from build123d import *

# Parameters (mm, degrees)
BOX023_W     = 2
BOX023_H     = 10
BOX023_DEPTH = 8.5
BOX025_W     = 6
BOX025_H     = 14
BOX025_DEPTH = 1


with BuildPart() as control_button_rec_c:
    # Box023 → Box023 (new body)
    with BuildSketch(Plane(origin=(57.3, 93.3, 9.6), x_dir=(1, 0, 0), z_dir=(0, 0, 1))):
        with Locations((1, 5)):
            Rectangle(BOX023_W, BOX023_H)
    extrude(amount=BOX023_DEPTH)


with BuildPart() as control_button_rec:
    # Box025 → Box025 (new body)
    with BuildSketch(Plane(origin=(55.3, 91.3, 9.6), x_dir=(1, 0, 0), z_dir=(0, 0, 1))):
        with Locations((3, 7)):
            Rectangle(BOX025_W, BOX025_H)
    extrude(amount=BOX025_DEPTH)

    # Fusion036: union control_button_rec_c
    add(control_button_rec_c.part)


solid = control_button_rec.part
The listing builds one solid part. Answer for the finished solid, in the listing's coordinates (mm). A direction names the side the tool comes from. Give positions to 0.01 mm unless a question says otherwise; leave off trailing zeros. Write each loop counter-clockwise with the first axis right and the second up, starting at its lowest first coordinate (ties: lowest second). Pieces come first, ordered by that corner, then holes.
Item 1: Section C-C, the plane z = 17.75 is taken. Write down the section's boundary in (x, y), plus the area to 3 significant figures.
Item 2: Section A-A, the plane y = 101 is taken. Write down the section's boundary in (x, z).
Item 3: Section B-B, the plane x = 58.2 is taken. Write down the section's boundary in (y, z).
Item 4: Which of the six approach directions +Z, -Z, +X, -X, +Y, -Y give full straight-line access (tool end or side, diameter ignored) to faces 1 (the flat face through (58, 93.3, 14)), 2 (the flat face through (58, 103.3, 14)), 3 (the flat face through (57.3, 98, 14)), 4 (the flat face through (59.3, 98, 14))?
Item 5: Section D-D, the plane y = 92 is taken. Write down the section's boundary in (x, z).
Item 6: Find the intervals of material crossed by line 1 along X through (y, z) = (101.5, 13); line 2 along Z through (x, y) = (59.4, 101.75); line 3 along Y through (x, z) = (59.15, 14), in increasing order.
Item 7: Flat-ended cylindrical pins translate along their axes: P1, Ø1.5, axis at x = 56.5, z = 15, coming from the -Y side; P2, Ø1, axis at y = 97.5, z = 15, coming from the +X side; P3, Ø1, axis at x = 58.5, z = 12.5, coming from the -Y side; P4, Ø1.5, axis at x = 58, z = 16, coming from the +Y side. Find the tip coordinate at first contact, or state that the pin passes through.
Completed:
1. outline: (57.3, 93.3) - (59.3, 93.3) - (59.3, 103.3) - (57.3, 103.3) - close
1. area: 20.0 mm2
2. outline: (55.3, 9.6) - (61.3, 9.6) - (61.3, 10.6) - (59.3, 10.6) - (59.3, 18.1) - (57.3, 18.1) - (57.3, 10.6) - (55.3, 10.6) - close
3. outline: (91.3, 9.6) - (105.3, 9.6) - (105.3, 10.6) - (103.3, 10.6) - (103.3, 18.1) - (93.3, 18.1) - (93.3, 10.6) - (91.3, 10.6) - close
4. face 1: +Z, +X, -X, -Y
4. face 2: +Z, +X, -X, +Y
4. face 3: +Z, -X, +Y, -Y
4. face 4: +Z, +X, +Y, -Y
5. outline: (55.3, 9.6) - (61.3, 9.6) - (61.3, 10.6) - (55.3, 10.6) - close
6. line 1: x = 57.3 to 59.3
6. line 2: z = 9.6 to 10.6
6. line 3: y = 93.3 to 103.3
7. P1: passes through
7. P2: stops at x = 59.3
7. P3: stops at y = 93.3
7. P4: stops at y = 103.3
